```python
from build123d import *

# Parameters (mm, degrees)
F1_DEPTH = 5
F2_R     = 1.6
F3_DEPTH = 3
F4_R     = 2


with BuildPart() as f1:
    # F0 (on Top) → F1 (new body)
    with BuildSketch(Plane.XY):
        Polygon((-48.657436, 0), (0, 0), (0, 12), (-2, 12), (-2, 2), (-22, 2), (-22, 8), (-48.657436, 8), (-60, 10), (-60, 8), (-48.657436, 6), (-26, 6), (-26, 2), (-48.657436, 2), (-60, 0), (-60, -2), align=None)
    extrude(amount=F1_DEPTH)

    # F2 (on face) → F3 (cut)
    with BuildSketch(Plane.YZ):
        with Locations((9, 2.5)):
            Circle(F2_R)
    extrude(amount=-F3_DEPTH, mode=Mode.SUBTRACT)

    # F4
    f4_edges = [f1.edges().sort_by_distance(p)[0] for p in [
        (-22, 8, 2.5),
    ]]
    fillet(f4_edges, radius=F4_R)


solid = f1.part
```
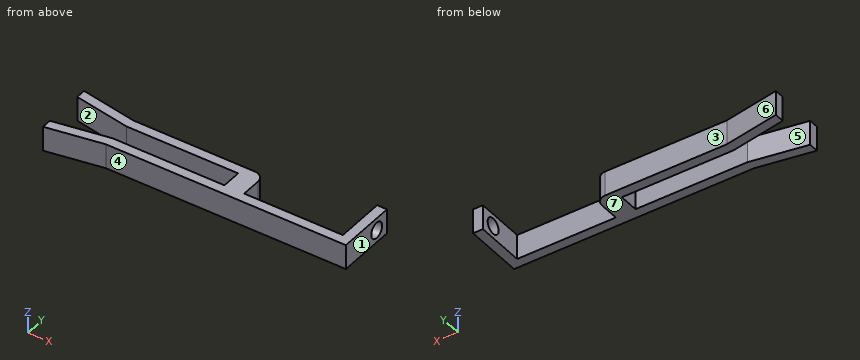
Read the model definition and answer for the solid it produces. Units are mm, in the model's axes. Face numbers are marked on the shaded views. A direction names the side the tool comes from. Round coordinates to 2 decimals unless told otherwise and drop trailing zeros. Write each loop counter-clockwise with the first axis right and the second up, starting at its lowest first coordinate (ties: lowest second). Pieces come first, ordered by that corner, then holes. Notation, with made-up numbers: (67, 43) - (105, 43) arc R23 ccw to (105, 71) - close; hole circle Ø5 at (-27.5, -18). An arc over 180 degrees is marked (long way). One line per item, written item: value.
Q1. Find section B-B (z = 2.5). Determine the outline of the cut face in (x, y).
The answers:
outline: (-60, -2) - (-48.66, 0) - (0, 0) - (0, 7.4) - (-2, 7.4) - (-2, 2) - (-22, 2) - (-22, 6) arc R2 ccw to (-24, 8) - (-48.66, 8) - (-60, 10) - (-60, 8) - (-48.66, 6) - (-26, 6) - (-26, 2) - (-48.66, 2) - (-60, 0) - close; (-2, 10.6) - (0, 10.6) - (0, 12) - (-2, 12) - close
Q2. Each of these flat-tipped pins is pushed along its axis until it touches: P1, Ø2, axis at x = -33.5, z = 3.5, coming from the -Y side; P2, Ø2, axis at y = 3.5, z = 2.5, coming from the -X side; P3, Ø1.5, axis at x = -31.5, z = 2, coming from the +Y side. Where does it stop, or does it pass through?
The answers:
P1: stops at y = 0
P2: stops at x = -26
P3: stops at y = 8
Q3. Find section C-C (x = -33.5). Determine the outline of the cut face in (y, z).
The answers:
outline: (0, 0) - (2, 0) - (2, 5) - (0, 5) - close; (6, 0) - (8, 0) - (8, 5) - (6, 5) - close
Q4. Which of the six approach directions +Z, -Z, +X, -X, +Y, -Y give full straight-line access (tool end or side, diameter ignored) to the marked faces 5, 6 and 7?
The answers:
face 5: +Z, -Z, -X
face 6: +Z, -Z, +Y
face 7: -Z, +X, -X, +Y, -Y
Q5. Find section D-D (y = 9). Determine the outline of the cut face in (x, z).
The answers:
outline: (-60, 0) - (-54.33, 0) - (-54.33, 5) - (-60, 5) - close; (-2, 0) - (0, 0) - (0, 0.9) - (-2, 0.9) - close; (-2, 4.1) - (0, 4.1) - (0, 5) - (-2, 5) - close
Q6. For a pull along Y with two mould halves and no side action, classify the marked faces 1, 2, 3 and 4 as pulls with the +Y half, pulls with the -Y half, needs draft (parallel to the pull), parting line crosses it, or undercut.
The answers:
face 1: needs draft
face 2: undercut
face 3: pulls with the +Y half
face 4: pulls with the -Y half
Q7. Find section A-A (y = 4.5). Determine the outline of the cut face in (x, z), and give its area (3 significant figures).
The answers:
outline: (-26, 0) - (-22, 0) - (-22, 5) - (-26, 5) - close; (-2, 0) - (0, 0) - (0, 5) - (-2, 5) - close
area: 30.0 mm2
Q8. Straight lines are drawn through the part: line 1 (X direction, y = 2.5, z = 1.85); line 2 (Y direction, x = -34, z = 2.2); line 3 (Z direction, x = -1.05, y = 9). For each, find the intervals that lie inside material, in ascending order. Write a range as from..to.
The answers:
line 1: x = -26..-22, -2..0
line 2: y = 0..2, 6..8
line 3: z = 0..0.9, 4.1..5
